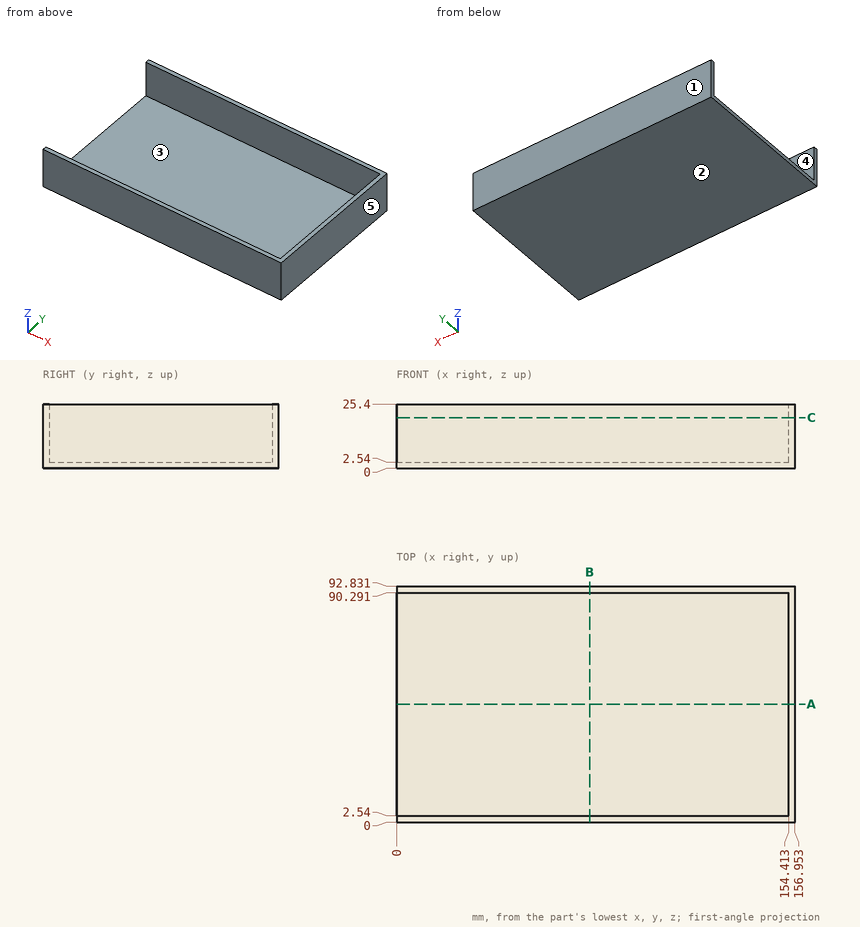
Part print with two shaded views. Sizes in mm from the minimum x, y, z corner. A direction names the side the tool comes from. Coordinates: 2 decimals unless noted, no trailing zeros. Order: outer loops, then holes, each group sorted by start corner. A loop starts at its lowest first (then second) coordinate and runs counter-clockwise, first axis right, second up. Notation, with made-up numbers: M 70.25,-24 L 115.25,-24 A18 ccw 115.25,-10 Z; hole C 27,48 d6. An arc over 180 degrees is marked long. One line per question, with ' | ' between items. Start each with the question number.
1. Wall check: line 1 along Y through (x, z) = (104, 19.5); line 2 along X through (y, z) = (62, 22.5); line 3 along Z through (x, y) = (71, 13). Give the ranges that are in metal, low to high. Write a range as [from, to].
2. Tool access for the marked faces 4 and 5: list every direction of +Z, -Z, +X, -X, +Y, -Y with a clear straight run to the whole face (end or side of a thin tool).
3. Flat gauge pins, fed straight in: P1, Ø11.5, axis at y = 63.5, z = 11.5, coming from the -X side; P2, Ø12, axis at x = 131.5, y = 22.5, coming from the +Z side. Where does each tip first touch, or does it go through?
4. Mould opens along Y. For the marked faces 1, 2 and 3 say: +Y half, -Y half, draft (parallel to the pull), parting line (faces both ways), or undercut.
5. Cut at B-B (x = 76). Write the cut outline in (y, z).
6. Cut at C-C (z = 20). Write the cut outline in (x, y).
7. Cut at A-A (y = 46.5). Write the cut outline in (x, z).
The answers:
1) line 1: y = [0, 2.54], [90.29, 92.83] | line 2: x = [154.41, 156.95] | line 3: z = [0, 2.54]
2) face 4: +Z, -X | face 5: +Z, -Z, +X, +Y, -Y
3) P1: stops at x = 154.41 | P2: stops at z = 2.54
4) face 1: +Y half | face 2: draft | face 3: undercut
5) outline: M 0,0 L 92.83,0 L 92.83,25.4 L 90.29,25.4 L 90.29,2.54 L 2.54,2.54 L 2.54,25.4 L 0,25.4 Z
6) outline: M 0,0 L 156.95,0 L 156.95,92.83 L 0,92.83 L 0,90.29 L 154.41,90.29 L 154.41,2.54 L 0,2.54 Z
7) outline: M 0,0 L 156.95,0 L 156.95,25.4 L 154.41,25.4 L 154.41,2.54 L 0,2.54 Z
